from build123d import *

# Parameters (mm, degrees)
SKETCH1_W           = 150
SKETCH1_H           = 150
BOSS_EXTRUDE1_DEPTH = 8
SKETCH3_W           = 150
SKETCH3_H           = 150
BOSS_EXTRUDE2_DEPTH = 8
SKETCH4_W           = 150
SKETCH4_H           = 150
SKETCH4_R           = 4.743192734
BOSS_EXTRUDE3_DEPTH = 8


with BuildPart() as part:
    # Sketch1 → Boss-Extrude1 (new body)
    with BuildSketch(Plane.XY):
        Rectangle(SKETCH1_W, SKETCH1_H)
    extrude(amount=BOSS_EXTRUDE1_DEPTH)

    # Sketch3 → Boss-Extrude2 (add)
    with BuildSketch(Plane(origin=(75, 0, 0), x_dir=(0, 0, -1), z_dir=(1, 0, 0))):
        with Locations((67.149717674, -0.182693133)):
            Rectangle(SKETCH3_W, SKETCH3_H)
    extrude(amount=BOSS_EXTRUDE2_DEPTH)

    # Sketch4 → Boss-Extrude3 (add)
    with BuildSketch(Plane.ZY.offset(75)):
        with Locations((-67, 0)):
            Rectangle(SKETCH4_W, SKETCH4_H)
        with Locations(Location((-83.382184019, 0.420229312, 0), (0, 0, 270))):
            Circle(SKETCH4_R, mode=Mode.SUBTRACT)
    extrude(amount=BOSS_EXTRUDE3_DEPTH)


solid = part.part
Can you work these out from the model? Positions are in its coordinate system, mm. A direction names the side the tool comes from. Coordinates: 2 decimals unless noted, no trailing zeros. Order: outer loops, then holes, each group sorted by start corner. A loop starts at its lowest first (then second) coordinate and runs counter-clockwise, first axis right, second up. Notation, with made-up numbers: (27.25, 53.5) - (53.25, 53.5) arc R3 ccw to (53.25, 57.5) - close; hole circle Ø2 at (12.25, 25.5). An arc over 180 degrees is marked (long way). Answer as a JSON object with one key per item and string values. Group by question number.
Q1. We'd pull the mould along X, two halves only. Please class faces 1 (the face through (-39, -75, 5)), 2 (the face through (83, 1, -66)), 3 (the face through (75, 1, -66)): +X half, -X half, draft (parallel to the pull), parting line (faces both ways), or undercut.
Q2. Will these pins go through, and if not, where does the flat tip stop? P1, Ø1.5, axis at x = -44.5, y = 11, coming from the -Z side; P2, Ø4, axis at x = -77.5, y = 27.5, coming from the -Z side; P3, Ø9, axis at x = 77, z = -33, coming from the +Y side.
Q3. Imagine slicing it at C-C (x = -26.5). Please give me the cut outline in (y, z), and give its area (3 significant figures).
Q4. On a 3-axis mill with a long thin cutter (end or side, diameter ignored), from which of +Z, -Z, +X, -X, +Y, -Y can I reach the whole of each face in a straight line? I mean faces 4 (the face through (-75, 1, -72)), 5 (the face through (-78.94, -1.77, -87.59)), 6 (the face through (79, -75.183, -66)), 7 (the face through (79, 74.817, -66)). Say none if no direction works.
Q5. Imagine slicing it at A-A (z = -45). Please give me the cut outline in (x, y), and give its area (3 significant figures).
Q6. I need wall thicknesses on line 1 (X direction, y = -38, z = -111); line 2 (Z direction, x = -39, y = 16). Which ranges of each line are inside material? Lowest first, please. Write a range as from..to.
Q7. Imagine slicing it at B-B (y = -58). Please give me the cut outline in (x, z).
Determined:
{
 "1": {"face 1": "draft", "face 2": "+X half", "face 3": "undercut"},
 "2": {"P1": "stops at z = 0", "P2": "stops at z = -142", "P3": "stops at y = 74.82"},
 "3": {"outline": "(-75, 0) - (75, 0) - (75, 8) - (-75, 8) - close", "area": "1,200 mm2"},
 "4": {"face 4": "-Z, +Y, -Y", "face 5": "-X", "face 6": "+Z, -Z, +X, -X, -Y", "face 7": "+Z, -Z, +X, +Y"},
 "5": {"outline": "(-83, -75) - (-75, -75) - (-75, 75) - (-83, 75) - close; (75, -75.18) - (83, -75.18) - (83, 74.82) - (75, 74.82) - close", "area": "2,400 mm2"},
 "6": {"line 1": "x = -83..-75, 75..83", "line 2": "z = 0..8"},
 "7": {"outline": "(-83, -142) - (-75, -142) - (-75, 0) - (75, 0) - (75, -142.15) - (83, -142.15) - (83, 7.85) - (75, 7.85) - (75, 8) - (-83, 8) - close"}
}
